from build123d import *

# Parameters (mm, degrees)
F0_W     = 152.4
F0_H     = 88.9
F0_R     = 16.51
F1_DEPTH = 12.7


with BuildPart() as f1:
    # F0 (on Top) → F1 (new body)
    with BuildSketch(Plane.XY):
        Rectangle(F0_W, F0_H)
        with Locations((-44.45, -12.7)):
            Circle(F0_R, mode=Mode.SUBTRACT)
        with Locations((44.45, -12.7)):
            Circle(F0_R, mode=Mode.SUBTRACT)
        with Locations((0, 12.7)):
            Circle(F0_R, mode=Mode.SUBTRACT)
    extrude(amount=-F1_DEPTH)


solid = f1.part
Geometry: final body of the model. Coordinates: model frame, mm. Coordinates: 2 decimals unless noted, no trailing zeros. Order: outer loops, then holes, each group sorted by start corner. A loop starts at its lowest first (then second) coordinate and runs counter-clockwise, first axis right, second up. Notation, with made-up numbers: M 79,49.25 L 93,49.25 A21 ccw 93,70.25 Z; hole C -7.75,75.25 d11. An arc over 180 degrees is marked long. One line per question, with ' | ' between items. Start each with the question number.
Item 1: Cut plane B-B, the plane x = -44.45. Return the cut outline in (y, z), then the cut area to 3 significant figures.
Item 2: Cut plane C-C, the plane z = -8.25. Return the cut outline in (x, y), then the cut area to 3 significant figures.
Item 3: Draft query along X for faces 1 (the flat face through (76.2, -1, -6)), 2 (the cylindrical face through (-29.199, -19.023, -6.261)), 3 (the flat face through (-1, -9, 0)), 4 (the cylindrical face through (8.88, 26.62, -6.26)). Return one class per face: released by +X, released by -X, zero draft, split by the parting line, or undercut.
Item 4: Cut plane D-D, the plane y = -12.7. Return the cut outline in (x, z).
Item 5: Ray query, probe 1 along Y at (x, z) = (-44.45, -6.75); probe 2 along X at (y, z) = (-22.5, -1.5); probe 3 along Y at (x, z) = (0, -5.75). Return the intervals inside material, ascending. Write a range as [from, to].
Item 6: Cut plane A-A, the plane y = 12.7. Return the cut outline in (x, z), then the cut area to 3 significant figures.
A:
1) outline: M -44.45,-12.7 L -29.21,-12.7 L -29.21,0 L -44.45,0 Z; M 3.81,-12.7 L 44.45,-12.7 L 44.45,0 L 3.81,0 Z | area: 710 mm2
2) outline: M -76.2,-44.45 L 76.2,-44.45 L 76.2,44.45 L -76.2,44.45 Z; hole C -44.45,-12.7 d33.02; hole C 0,12.7 d33.02; hole C 44.45,-12.7 d33.02 | area: 11,000 mm2
3) face 1: released by +X | face 2: undercut | face 3: zero draft | face 4: undercut
4) outline: M -76.2,-12.7 L -60.96,-12.7 L -60.96,0 L -76.2,0 Z; M -27.94,-12.7 L 27.94,-12.7 L 27.94,0 L -27.94,0 Z; M 60.96,-12.7 L 76.2,-12.7 L 76.2,0 L 60.96,0 Z
5) probe 1: y = [-44.45, -29.21], [3.81, 44.45] | probe 2: x = [-76.2, -57.74], [-31.16, 31.16], [57.74, 76.2] | probe 3: y = [-44.45, -3.81], [29.21, 44.45]
6) outline: M -76.2,-12.7 L -16.51,-12.7 L -16.51,0 L -76.2,0 Z; M 16.51,-12.7 L 76.2,-12.7 L 76.2,0 L 16.51,0 Z | area: 1,520 mm2
